Can you work these out from the model? Positions are in its coordinate system, mm. A direction names the side the tool comes from. Give positions to 0.01 mm unless a question says otherwise; leave off trailing zeros. Write each loop counter-clockwise with the first axis right and the second up, starting at its lowest first coordinate (ties: lowest second). Pieces come first, ordered by that corner, then holes. Notation, with made-up numbers: M 56.5,-29.75 L 87.5,-29.75 A15 ccw 87.5,-4.75 Z; hole C 32,66.5 d3. An arc over 180 degrees is marked long. Use CSV: the item, a comma, the result in double quotes. Start each with the question number.
from build123d import *

# Parameters (mm, degrees)
SKETCH1_R           = 4
BOSS_EXTRUDE1_DEPTH = 15.24
SKETCH2_W           = 25.4
SKETCH2_H           = 11.5697
CUT_EXTRUDE1_DEPTH  = 26.4
SKETCH3_W           = 10.75005279
SKETCH3_H           = 13.530974344
CUT_EXTRUDE2_DEPTH  = 26.4
SKETCH4_R           = 4
CUT_EXTRUDE3_DEPTH  = 41.64


with BuildPart() as part:
    # Sketch1 → Boss-Extrude1 (new body)
    with BuildSketch(Plane.XY):
        with BuildLine():
            Line((0, 12.7), (27.94, 12.7))
            Line((27.94, 12.7), (27.94, -12.7))
            Line((27.94, -12.7), (0, -12.7))
            ThreePointArc((0, -12.7), (-12.7, 0), (0, 12.7))
        make_face()
        Circle(SKETCH1_R, mode=Mode.SUBTRACT)
    extrude(amount=BOSS_EXTRUDE1_DEPTH)

    # Sketch2 → Cut-Extrude1 (cut, through all)
    with BuildSketch(Plane(origin=(0, 12.7, 0), x_dir=(1, 0, 0), z_dir=(0, 1, 0))):
        with Locations((0, -7.62)):
            Rectangle(SKETCH2_W, SKETCH2_H)
    extrude(amount=-CUT_EXTRUDE1_DEPTH, mode=Mode.SUBTRACT)

    # Sketch3 → Cut-Extrude2 (cut, through all)
    with BuildSketch(Plane(origin=(0, 12.7, 0), x_dir=(1, 0, 0), z_dir=(0, 1, 0))):
        with Locations((22.053049583, -7.62)):
            Rectangle(SKETCH3_W, SKETCH3_H)
    extrude(amount=-CUT_EXTRUDE2_DEPTH, mode=Mode.SUBTRACT)

    # Sketch4 → Cut-Extrude3 (cut, through all)
    with BuildSketch(Plane(origin=(27.94, 0, 0), x_dir=(0, 0, -1), z_dir=(1, 0, 0))):
        with Locations((-7.62, 0)):
            Circle(SKETCH4_R)
    extrude(amount=-CUT_EXTRUDE3_DEPTH, mode=Mode.SUBTRACT)


solid = part.part
(1) I want a section at A-A (z = 7.62). Write out the boundary of the cut face in (x, y).
(2) I want a section at C-C (y = 0). Write out the boundary of the cut face in (x, z), and give its area (3 significant figures).
(3) I want a section at D-D (y = -8.5). Write out the boundary of the cut face in (x, z).
(4) I want a section at B-B (x = 11). Write out the boundary of the cut face in (y, z).
(5) Which directions (+Z, -Z, +X, -X, +Y, -Y) give clear straight access to the entire face, cutting with the end or side of a thin tool? Please do faces 1 (the face through (16.678, 3, 11)), 2 (the face through (-0.867, -3.905, 14.31)), 3 (the face through (5, 0, 1.835)).
(6) Will this pin go through, and if not, where does the flat tip stop? pin 1 Ø4 at (y, z) = (-4.5, 8.5) entering from -X.
(7) Please list where these lines run through material, in increasing order: L1, parallel to Z at x = 19.5, y = 2.75; L2, parallel to X at y = 2, z = 3.75; L3, parallel to Z at x = -7.5, y = -2.25. Write a range as [from, to].
(8) Thinking about a two-plate mould opening in Z: for faces 4 (the face through (8, 0, 15.24)), 5 (the face through (-0.867, -3.905, 0.905)), 6 (the face through (27.428, 3, 11)), which applies, released by +Z, released by -Z, zero draft, split by the parting line, or undercut?
Geometry results:
1,outline,"M 12.7,-12.7 L 16.68,-12.7 L 16.68,-4 L 12.7,-4 Z; M 12.7,4 L 16.68,4 L 16.68,12.7 L 12.7,12.7 Z; M 27.43,-12.7 L 27.94,-12.7 L 27.94,-4 L 27.43,-4 Z; M 27.43,4 L 27.94,4 L 27.94,12.7 L 27.43,12.7 Z"
2,outline,"M -12.7,0 L -4,0 L -4,1.84 L -12.7,1.84 Z; M -12.7,13.4 L -4,13.4 L -4,15.24 L -12.7,15.24 Z; M 4,0 L 27.94,0 L 27.94,3.62 L 27.43,3.62 L 27.43,0.85 L 16.68,0.85 L 16.68,3.62 L 12.7,3.62 L 12.7,1.84 L 4,1.84 Z; M 4,13.4 L 12.7,13.4 L 12.7,11.62 L 16.68,11.62 L 16.68,14.39 L 27.43,14.39 L 27.43,11.62 L 27.94,11.62 L 27.94,15.24 L 4,15.24 Z"
2,area,"115 mm2"
3,outline,"M -9.44,0 L 27.94,0 L 27.94,15.24 L -9.44,15.24 L -9.44,13.4 L 12.7,13.4 L 12.7,1.84 L -9.44,1.84 Z; hole M 16.68,0.85 L 27.43,0.85 L 27.43,14.39 L 16.68,14.39 Z"
4,outline,"M -12.7,0 L 12.7,0 L 12.7,1.84 L -12.7,1.84 Z; M -12.7,13.4 L 12.7,13.4 L 12.7,15.24 L -12.7,15.24 Z"
5,face 1,"+Y, -Y"
5,face 2,"+Z, -Z"
5,face 3,"-X, +Y, -Y"
6,pin 1,"stops at x = 12.7"
7,L1,"z = [0, 0.85], [14.39, 15.24]"
7,L2,"x = [12.7, 16.68], [27.43, 27.94]"
7,L3,"z = [0, 1.84], [13.4, 15.24]"
8,face 4,"released by +Z"
8,face 5,"zero draft"
8,face 6,"undercut"
